```python
from build123d import *

# Parameters (mm, degrees)
BOSS_EXTRUDE1_REACH                             = 4.654
BOSS_EXTRUDE1_DIRECTION_2_REACH                 = 4.654
CSK_FOR_M2_RAISED_CROSS_HEAD_SCREW1_D           = 2.6
CSK_FOR_M2_RAISED_CROSS_HEAD_SCREW1_CSINK_D     = 4.6
CSK_FOR_M2_RAISED_CROSS_HEAD_SCREW1_CSINK_ANGLE = 92


with BuildPart() as part:
    # Sketch4 → Revolve3 (revolve)
    with BuildSketch(Plane(origin=(0, 0, 0), x_dir=(0, 0, -1), z_dir=(1, 0, 0))):
        with BuildLine():
            Line((-2.6543, -39.6621), (-1.7653, -39.6621))
            ThreePointArc((-1.7653, -39.6621), (0, -37.8968), (1.7653, -39.6621))
            Line((1.7653, -39.6621), (2.6543, -39.6621))
            Line((2.6543, -39.6621), (2.6543, -37.0078))
            Line((2.6543, -37.0078), (-2.6543, -37.0078))
            Line((-2.6543, -37.0078), (-2.6543, -39.6621))
        make_face()
    revolve(axis=Axis((0, 0, 1.7653), (0, 0, -1)))

    # Boss-Extrude1: up to this face of the body (flat: up to its plane)
    boss_extrude1_end = Plane(part.part.faces().sort_by_distance((0, 38.540286405, -2.6543))[0])
    # Sketch5 → Boss-Extrude1 (add, up to the picked face)
    with BuildSketch(Plane.XY, mode=Mode.PRIVATE) as boss_extrude1_sk1:
        with BuildLine():
            ThreePointArc((2.978912783, -11.636990203), (10.402888866, -6.006110687), (11.56738553, 3.238680956))
            ThreePointArc((11.56738553, 3.238680956), (26.749196364, 4.65193852), (37.371776023, -6.286319044))
            ThreePointArc((37.371776023, -6.286319044), (37.895229039, -0.345059896), (37.48005165, 5.604746073))
            add(Edge.make_bspline(
                [(15.506400774, 8.952624661), (27.141070528, 11.852195949), (37.48005165, 5.604746073)],
                knots=[0, 0, 0, 1, 1, 1], degree=2))
            add(Edge.make_bspline(
                [(15.506400774, 8.952624661), (23.43091271, 17.496942665), (24.189816075, 29.172251345)],
                knots=[0, 0, 0, 1, 1, 1], degree=2))
            ThreePointArc((24.189816075, 29.172251345), (18.982008892, 32.800164461), (13.241776023, 35.508066943))
            ThreePointArc((13.241776023, 35.508066943), (17.403295117, 20.839514322), (8.588472748, 8.398309247))
            ThreePointArc((8.588472748, 8.398309247), (0, 12.012221374), (-8.588472748, 8.398309247))
            ThreePointArc((-8.588472748, 8.398309247), (-17.403295117, 20.839514322), (-13.241776023, 35.508066943))
            ThreePointArc((-13.241776023, 35.508066943), (-18.231527824, 33.22316727), (-22.83893963, 30.241532482))
            add(Edge.make_bspline(
                [(-15.506400774, 8.952624661), (-24.330033969, 17.722070983), (-22.83893963, 30.241532482)],
                knots=[0, 0, 0, 1, 1, 1], degree=2))
            add(Edge.make_bspline(
                [(-15.506400774, 8.952624661), (-27.512780663, 12.209392), (-37.609405193, 4.658335674)],
                knots=[0, 0, 0, 1, 1, 1], degree=2))
            ThreePointArc((-37.609405193, 4.658335674), (-37.887870762, -0.822617389), (-37.371776023, -6.286319044))
            ThreePointArc((-37.371776023, -6.286319044), (-26.749196364, 4.65193852), (-11.56738553, 3.238680956))
            ThreePointArc((-11.56738553, 3.238680956), (-10.402888866, -6.006110687), (-2.978912783, -11.636990203))
            ThreePointArc((-2.978912783, -11.636990203), (-9.345901247, -25.491452842), (-24.13, -29.221747898))
            ThreePointArc((-24.13, -29.221747898), (-19.656342938, -32.400549881), (-14.770465564, -34.899868156))
            add(Edge.make_bspline(
                [(0, -17.905249322), (-3.182746695, -29.931462983), (-14.770465564, -34.899868156)],
                knots=[0, 0, 0, 1, 1, 1], degree=2))
            add(Edge.make_bspline(
                [(0, -17.905249322), (3.182746695, -29.931462983), (14.770465564, -34.899868156)],
                knots=[0, 0, 0, 1, 1, 1], degree=2))
            ThreePointArc((14.770465564, -34.899868156), (19.656342938, -32.400549881), (24.13, -29.221747898))
            ThreePointArc((24.13, -29.221747898), (9.345901247, -25.491452842), (2.978912783, -11.636990203))
        make_face()
    boss_extrude1_tool1 = split(extrude(boss_extrude1_sk1.sketch, amount=-BOSS_EXTRUDE1_REACH, mode=Mode.PRIVATE), bisect_by=boss_extrude1_end, keep=Keep.BOTH, mode=Mode.PRIVATE)
    add(boss_extrude1_tool1.solids().sort_by_distance((0.196494, 0.141193, 0))[0])

    # Boss-Extrude1 direction 2: up to this face of the body (flat: up to its plane)
    boss_extrude1_direction_2_end = Plane(part.part.faces().sort_by_distance((0, 38.129613595, 2.6543))[0])
    # Sketch5 → Boss-Extrude1 direction 2 (add, up to the picked face)
    with BuildSketch(Plane.XY, mode=Mode.PRIVATE) as boss_extrude1_direction_2_sk1:
        with BuildLine():
            ThreePointArc((2.978912783, -11.636990203), (10.402888866, -6.006110687), (11.56738553, 3.238680956))
            ThreePointArc((11.56738553, 3.238680956), (26.749196364, 4.65193852), (37.371776023, -6.286319044))
            ThreePointArc((37.371776023, -6.286319044), (37.895229039, -0.345059896), (37.48005165, 5.604746073))
            add(Edge.make_bspline(
                [(15.506400774, 8.952624661), (27.141070528, 11.852195949), (37.48005165, 5.604746073)],
                knots=[0, 0, 0, 1, 1, 1], degree=2))
            add(Edge.make_bspline(
                [(15.506400774, 8.952624661), (23.43091271, 17.496942665), (24.189816075, 29.172251345)],
                knots=[0, 0, 0, 1, 1, 1], degree=2))
            ThreePointArc((24.189816075, 29.172251345), (18.982008892, 32.800164461), (13.241776023, 35.508066943))
            ThreePointArc((13.241776023, 35.508066943), (17.403295117, 20.839514322), (8.588472748, 8.398309247))
            ThreePointArc((8.588472748, 8.398309247), (0, 12.012221374), (-8.588472748, 8.398309247))
            ThreePointArc((-8.588472748, 8.398309247), (-17.403295117, 20.839514322), (-13.241776023, 35.508066943))
            ThreePointArc((-13.241776023, 35.508066943), (-18.231527824, 33.22316727), (-22.83893963, 30.241532482))
            add(Edge.make_bspline(
                [(-15.506400774, 8.952624661), (-24.330033969, 17.722070983), (-22.83893963, 30.241532482)],
                knots=[0, 0, 0, 1, 1, 1], degree=2))
            add(Edge.make_bspline(
                [(-15.506400774, 8.952624661), (-27.512780663, 12.209392), (-37.609405193, 4.658335674)],
                knots=[0, 0, 0, 1, 1, 1], degree=2))
            ThreePointArc((-37.609405193, 4.658335674), (-37.887870762, -0.822617389), (-37.371776023, -6.286319044))
            ThreePointArc((-37.371776023, -6.286319044), (-26.749196364, 4.65193852), (-11.56738553, 3.238680956))
            ThreePointArc((-11.56738553, 3.238680956), (-10.402888866, -6.006110687), (-2.978912783, -11.636990203))
            ThreePointArc((-2.978912783, -11.636990203), (-9.345901247, -25.491452842), (-24.13, -29.221747898))
            ThreePointArc((-24.13, -29.221747898), (-19.656342938, -32.400549881), (-14.770465564, -34.899868156))
            add(Edge.make_bspline(
                [(0, -17.905249322), (-3.182746695, -29.931462983), (-14.770465564, -34.899868156)],
                knots=[0, 0, 0, 1, 1, 1], degree=2))
            add(Edge.make_bspline(
                [(0, -17.905249322), (3.182746695, -29.931462983), (14.770465564, -34.899868156)],
                knots=[0, 0, 0, 1, 1, 1], degree=2))
            ThreePointArc((14.770465564, -34.899868156), (19.656342938, -32.400549881), (24.13, -29.221747898))
            ThreePointArc((24.13, -29.221747898), (9.345901247, -25.491452842), (2.978912783, -11.636990203))
        make_face()
    boss_extrude1_direction_2_tool1 = split(extrude(boss_extrude1_direction_2_sk1.sketch, amount=BOSS_EXTRUDE1_DIRECTION_2_REACH, mode=Mode.PRIVATE), bisect_by=boss_extrude1_direction_2_end, keep=Keep.BOTH, mode=Mode.PRIVATE)
    add(boss_extrude1_direction_2_tool1.solids().sort_by_distance((0.196494, 0.141193, 0))[0])

    # CSK for M2 Raised Cross Head Screw1 (through all)
    with Locations(Plane(origin=(0, 0, -2.6543), x_dir=(-1, 0, 0), z_dir=(0, 0, -1))):
        with Locations((0, 0)):
            CounterSinkHole(CSK_FOR_M2_RAISED_CROSS_HEAD_SCREW1_D / 2, CSK_FOR_M2_RAISED_CROSS_HEAD_SCREW1_CSINK_D / 2, counter_sink_angle=CSK_FOR_M2_RAISED_CROSS_HEAD_SCREW1_CSINK_ANGLE)


solid = part.part
```
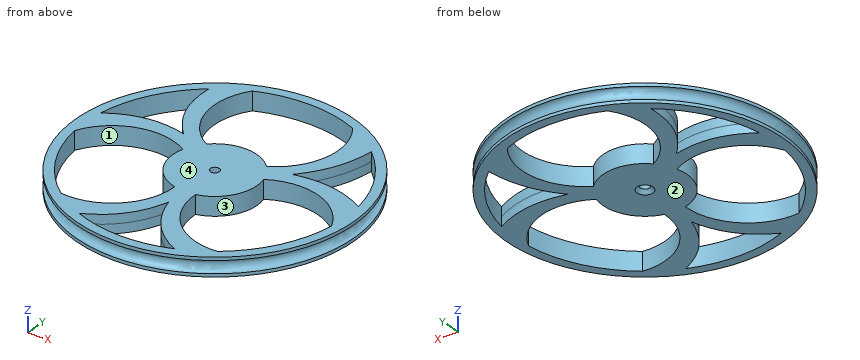
Build history of the part. All positions in model axes, mm. Face numbers are marked on the shaded views. A direction names the side the tool comes from. Give positions to 0.01 mm unless a question says otherwise; leave off trailing zeros. Loops run counter-clockwise (first coordinate to the right, second up) from the corner with the lowest first, then second, coordinate; pieces in that order, holes last. Notation, with made-up numbers: (18, 4.5) - (47, 4.5) arc R13 ccw to (47, 28.5) - close; hole circle Ø8 at (60, 61.5). An arc over 180 degrees is marked (long way). Use a Markdown table: item, result.
(1) Wall check: line 1 along Y through (x, z) = (-26.5, 0.4); line 2 along X through (y, z) = (-9, -2); line 3 along Y through (x, z) = (-19.5, 2.3). Give the ranges that are in metal, low to high.
Taken from the geometry:
| item | result |
|---|---|
| line 1 | -27.16 to -25.83, 4.74 to 9.6, 25.83 to 27.16 |
| line 2 | -38.63 to -35.9, -7.96 to 7.96, 35.9 to 38.63 |
| line 3 | -34.54 to -29.53, 5.71 to 9.74, 13.93 to 34.54 |
(2) Band-saw the part on A-A (y = 0). Give the cut face in (x, z), and give its area (3 significant figures).
Taken from the geometry:
| item | result |
|---|---|
| outline | (-39.66, -2.65) - (-33.67, -2.65) - (-33.67, 2.65) - (-39.66, 2.65) - (-39.66, 1.77) arc R1.77 cw to (-39.66, -1.77) - close; (-12.01, -2.65) - (-2.3, -2.65) - (-1.3, -1.69) - (-1.3, 2.65) - (-12.01, 2.65) - close; (1.3, -1.69) - (2.3, -2.65) - (12.01, -2.65) - (12.01, 2.65) - (1.3, 2.65) - close; (33.67, -2.65) - (39.66, -2.65) - (39.66, -1.77) arc R1.77 cw to (39.66, 1.77) - (39.66, 2.65) - (33.67, 2.65) - close |
| area | 167 mm2 |
(3) Drop flat-ended pins along their axis: pin 1 Ø1 at (y, z) = (22, -2) entering from +X; pin 2 Ø3 at (x, z) = (26.5, -2) entering from -Y. Give the stop position or say it passes through.
Taken from the geometry:
| item | result |
|---|---|
| pin 1 | x = 33.33 |
| pin 2 | y = -30.79 |
(4) Band-saw the part on B-B (x = 31). Give the number of separate pieces and of enclosed holes in the cut face, and give its area (3 significant figures).
Taken from the geometry:
| item | result |
|---|---|
| separate pieces | 3 |
| enclosed holes | 0 |
| area | 64.8 mm2 |
(5) Which spindle directions (+Z, -Z, +X, -X, +Y, -Y) get a long thin tool onto all of the face, cutting with end or side? Do the marked faces 3 and 4. Say none if no direction does.
Taken from the geometry:
| item | result |
|---|---|
| face 3 | +Z, -Z |
| face 4 | +Z, +X, -X, +Y, -Y |
(6) Pull direction Y, two halves, no side cores. Call the marked faces 1 and 2: +Y half, -Y half, draft (parallel to the pull), parting line (faces both ways), or undercut.
Taken from the geometry:
| item | result |
|---|---|
| face 1 | undercut |
| face 2 | draft |
